Build history of the part. All positions in model axes, mm. A direction names the side the tool comes from. Round coordinates to 2 decimals unless told otherwise and drop trailing zeros. Write each loop counter-clockwise with the first axis right and the second up, starting at its lowest first coordinate (ties: lowest second). Pieces come first, ordered by that corner, then holes. Notation, with made-up numbers: (14.25, -15.5) -> (51.25, -15.5) arc R22 ccw to (51.25, 16.5) -> close; hole circle Ø6 at (16.25, -1). An arc over 180 degrees is marked (long way). One line per question, with ' | ' between items.
Autodesk Inventor part; units mm, degrees
ref_plane "YZ Plane" through (0, 0, 0) normal (1, 0, 0) x (0, 1, 0)
ref_plane "XZ Plane" through (0, 0, 0) normal (0, 1, 0) x (-1, 0, 0)
ref_plane "XY Plane" through (0, 0, 0) normal (0, 0, 1) x (1, 0, 0)
sketch "Sketch1" plane through (0, 0, 0) normal (0, 0, 1) x (1, 0, 0)
  line L0 (0, 0) -> (25.4, 0)
  line L1 (25.4, 0) -> (25.4, 25.4)
  line L2 (25.4, 25.4) -> (0, 25.4)
  line L3 (0, 25.4) -> (0, 0)
  dimension "d0" = 25.4
  dimension "d1" = 25.4
extrude "Extrusion1" add sketch "Sketch1" along normal blind 2.54
sketch "Sketch2" plane through (0, 0, 2.54) normal (0, 0, 1) x (1, 0, 0)
  circle A0 centre (12.7, 12.7) radius 5.969
  line L0 (25.4, 25.4) -> (0, 25.4)
  line L1 (25.4, 0) -> (25.4, 25.4)
  point P0 (0, 0)
  dimension "d4" = 12.7
  dimension "d5" = 12.7
  dimension "d8" = 11.938
extrude "Extrusion2" cut sketch "Sketch2" against normal blind 2.54
sketch "Sketch3" plane through (0, 0, 0) normal (0, 0, -1) x (-1, 0, 0)
  line L0 (-18.796, 18.796) -> (-6.604, 18.796)
  line L1 (-6.604, 18.796) -> (-6.604, 6.604)
  line L2 (-6.604, 6.604) -> (-18.796, 6.604)
  line L3 (-18.796, 6.604) -> (-18.796, 18.796)
  line L4 (-25.4, 25.4) -> (0, 25.4)
  line L5 (0, 25.4) -> (0, 0)
  line L6 (-6.604, 13.97) -> (-5.334, 13.97)
  line L7 (-5.334, 13.97) -> (-5.334, 11.43)
  line L8 (-5.334, 11.43) -> (-6.604, 11.43)
  line L9 (-6.604, 11.43) -> (-6.604, 13.97)
  line L10 (-18.796, 13.97) -> (-20.066, 13.97)
  line L11 (-20.066, 13.97) -> (-20.066, 11.43)
  line L12 (-20.066, 11.43) -> (-18.796, 11.43)
  line L13 (-18.796, 11.43) -> (-18.796, 13.97)
  dimension "d9" = 12.192
  dimension "d10" = 12.192
  dimension "d11" = 6.604
  dimension "d12" = 6.604
  dimension "d13" = 1.27
  dimension "d14" = 1.27
  dimension "d15" = 2.54
  dimension "d16" = 11.43
  dimension "d17" = 2.54
extrude "Extrusion3" add sketch "Sketch3" along normal blind 7.62 contours L3 L12 L11 L10 | L6 L7 L8 L1
sketch "Sketch4" plane through (18.796, 11.43, 0) normal (0, -1, 0) x (1, 0, 0)
  line L0 (0, -7.62) -> (1.27, -7.62)
  line L1 (1.27, -7.62) -> (-1.27, -7.62)
  line L2 (-1.27, -7.62) -> (-1.27, -8.89)
  line L3 (-1.27, -8.89) -> (1.27, -8.89)
  line L4 (1.27, -8.89) -> (1.27, -7.62)
  line L5 (-1.27, -7.62) -> (0, -8.89)
  line L6 (-12.192, -7.62) -> (-13.462, -7.62)
  line L7 (-13.462, -7.62) -> (-10.922, -7.62)
  line L8 (-10.922, -7.62) -> (-10.922, -8.89)
  line L9 (-10.922, -8.89) -> (-13.462, -8.89)
  line L10 (-13.462, -8.89) -> (-13.462, -7.62)
  line L11 (-10.922, -7.62) -> (-12.192, -8.89)
  point P0 (-18.796, 0)
  dimension "d20" = 1.27
  dimension "d21" = 2.54
  dimension "d22" = 2.54
  dimension "d23" = 1.27
extrude "Extrusion4" add sketch "Sketch4" against normal blind 2.54 contours L0 L4 L3 L5 L1 | L7 L11 L9 L10 L6
sketch "Sketch5" plane through (18.796, 11.43, 0) normal (0, -1, 0) x (1, 0, 0)
  line L0 (6.604, 0) -> (-18.796, 0)
  line L1 (0.508, -5.715) -> (-12.7, -5.715)
  line L2 (-12.7, -5.715) -> (-12.7, 0)
  line L3 (-12.7, 0) -> (0.508, 0)
  line L4 (0.508, 0) -> (0.508, -5.715)
  line L5 (-13.462, 0) -> (-13.462, -8.89)
  dimension "d26" = 13.208
  dimension "d27" = 0.762
  dimension "d28" = 5.715
extrude "Extrusion5" cut sketch "Sketch5" against normal blind 2.54
chamfer "Chamfer1" distance 0.508 angle 45 2 edges at (6.604, 12.7, -5.715) (18.796, 12.7, -5.715)
properties part number "TestButtonClip"
(1) Mould opens along X. For faces 1 (the flat face through (5.8, 13.97, -5.4)), 2 (the flat face through (6.604, 13, -7)), 3 (the flat face through (25.4, 13, 1)) say: pulls with the +X half, pulls with the -X half, needs draft (parallel to the pull), parting line crosses it, or undercut.
Calculated:
face 1: needs draft | face 2: undercut | face 3: pulls with the +X half
(2) Wall check: line 1 (Y direction, x = 12.7, z = 1.5); line 2 (Z direction, x = 3.5, y = 11); line 3 (Y direction, x = 19.5, z = -4.5). Give the ranges that are in metal, low to high. Write a range as from..to.
Calculated:
line 1: 0..6.73, 18.67..25.4 | line 2: 0..2.54 | line 3: 11.43..13.97
(3) Slice it at A-A (x = 12.7). Write the cut outline in (y, z), then the cut area to 3 significant figures.
Calculated:
outline: (0, 0) -> (6.73, 0) -> (6.73, 2.54) -> (0, 2.54) -> close; (18.67, 0) -> (25.4, 0) -> (25.4, 2.54) -> (18.67, 2.54) -> close | area: 34.2 mm2
(4) Slice it at D-D (y = 21.5). Write the cut outline in (x, z).
Calculated:
outline: (0, 0) -> (25.4, 0) -> (25.4, 2.54) -> (0, 2.54) -> close
(5) Drop flat-ended pins along their axis: pin 1 (3 mm diameter, centred on x = 19.5, z = -4, fed in from +Y); pin 2 (3 mm diameter, centred on y = 12.5, z = -5.5, fed in from -X); pin 3 (0.8 mm diameter, centred on y = 13, z = -6.5, fed in from +X); pin 4 (6 mm diameter, centred on y = 7, z = 1, fed in from -X). Give the stop position or say it passes through.
Calculated:
pin 1: y = 13.97 | pin 2: x = 5.33 | pin 3: x = 20.07 | pin 4: x = 0
(6) Slice it at B-B (z = -2.5). Write the cut outline in (x, y), then the cut area to 3 significant figures.
Calculated:
outline: (5.33, 11.43) -> (6.1, 11.43) -> (6.1, 13.97) -> (5.33, 13.97) -> close; (19.3, 11.43) -> (20.07, 11.43) -> (20.07, 13.97) -> (19.3, 13.97) -> close | area: 3.87 mm2
(7) 3-axis set-ups, long thin cutter, end or side, ignore diameter. For faces 4 (the flat face through (5.7, 11.43, -5.4)), 5 (the flat face through (18.152, 12.682, -8.246)), 6 (the flat face through (19.6, 13.97, -5.4)), 7 (the flat face through (18.796, 13, -7)): which of +Z, -Z, +X, -X, +Y, -Y reach the whole face in a straight line?
Calculated:
face 4: -Z, +X, -X, -Y | face 5: -Z, +Y, -Y | face 6: -Z, +X, -X, +Y | face 7: +Y, -Y
